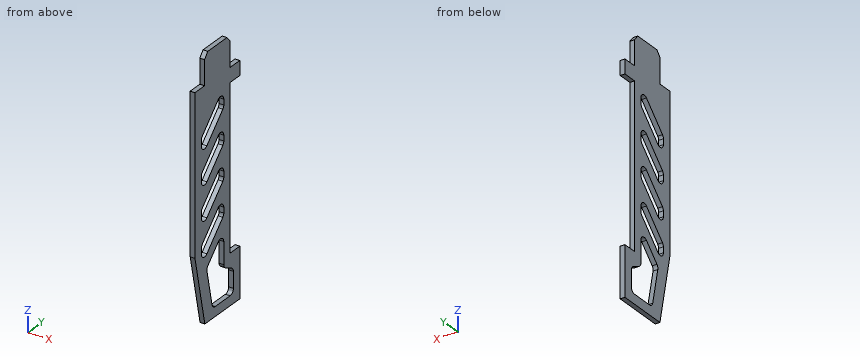
```python
from build123d import *

# Parameters (mm, degrees)
SKIZZE1_W                       = 237.5
SKIZZE1_H                       = 70
AUFSATZ_LINEAR_AUSTRAGEN1_DEPTH = 5
SCHNITT_LINEAR_AUSTRAGEN1_DEPTH = 248.651468802
SKIZZE3_W                       = 170
SKIZZE3_H                       = 15
SCHNITT_LINEAR_AUSTRAGEN2_DEPTH = 5
SCHNITT_LINEAR_AUSTRAGEN3_DEPTH = 248.651468802
VERRUNDUNG1_R                   = 5
LASCHENASE_DEPTH                = 5


with BuildPart() as part:
    # Skizze1 → Aufsatz-Linear austragen1 (new body)
    with BuildSketch(Plane(origin=(0, 0, 0), x_dir=(0, 0, -1), z_dir=(1, 0, 0))):
        with Locations((118.75, 35)):
            Rectangle(SKIZZE1_W, SKIZZE1_H)
    extrude(amount=AUFSATZ_LINEAR_AUSTRAGEN1_DEPTH)

    # Skizze2 → Schnitt-Linear austragen1 (cut, through all)
    with BuildSketch(Plane(origin=(5, 0, 0), x_dir=(0, 0, -1), z_dir=(1, 0, 0))):
        Polygon((165, 0), (237.5, 15.410350721), (237.5, 0), align=None)
    extrude(amount=-SCHNITT_LINEAR_AUSTRAGEN1_DEPTH, mode=Mode.SUBTRACT)

    # Skizze3 → Schnitt-Linear austragen2 (cut)
    with BuildSketch(Plane(origin=(5, 0, 0), x_dir=(0, 0, -1), z_dir=(1, 0, 0))):
        with Locations((100, 62.5)):
            Rectangle(SKIZZE3_W, SKIZZE3_H)
    extrude(amount=-SCHNITT_LINEAR_AUSTRAGEN2_DEPTH, mode=Mode.SUBTRACT)

    # Skizze4 → Schnitt-Linear austragen3 (cut, through all)
    with BuildSketch(Plane(origin=(5, 0, 0), x_dir=(0, 0, -1), z_dir=(1, 0, 0))):
        Polygon((15, 45), (50, 10), (70, 10), (35, 45), align=None)
        Polygon((50.884510848, 45), (70.884510848, 45), (105.884510848, 10), (85.884510848, 10), align=None)
        Polygon((86.769021696, 45), (106.769021696, 45), (141.769021696, 10), (121.769021696, 10), align=None)
        Polygon((122.653532545, 45), (142.653532545, 45), (177.653532545, 10), (157.653532545, 10), align=None)
        Polygon((227.5, 60), (227.5, 27.5), (183.622185543, 18.173482625), (156.795668168, 45), (195, 45), (202.5, 60), align=None)
    extrude(amount=-SCHNITT_LINEAR_AUSTRAGEN3_DEPTH, mode=Mode.SUBTRACT)

    # Verrundung1
    verrundung1_edges = [part.edges().sort_by_distance(p)[0] for p in [
        (2.5, 60, -202.5),
        (2.5, 60, -227.5),
        (2.5, 27.5, -227.5),
        (2.5, 18.173482625, -183.622185543),
        (2.5, 45, -156.795668168),
        (2.5, 45, -195),
        (2.5, 10, -85.884510848),
        (2.5, 45, -50.884510848),
        (2.5, 45, -70.884510848),
        (2.5, 10, -105.884510848),
        (2.5, 10, -157.653532545),
        (2.5, 45, -122.653532545),
        (2.5, 45, -142.653532545),
        (2.5, 10, -177.653532545),
        (2.5, 10, -121.769021696),
        (2.5, 45, -86.769021696),
        (2.5, 45, -106.769021696),
        (2.5, 10, -141.769021696),
        (2.5, 45, -15),
        (2.5, 45, -35),
        (2.5, 10, -70),
        (2.5, 10, -50),
    ]]
    fillet(verrundung1_edges, radius=VERRUNDUNG1_R)

    # Skizze5 → LascheNase (add)
    with BuildSketch(Plane(origin=(5, 0, 0), x_dir=(0, 0, -1), z_dir=(1, 0, 0))):
        Polygon((0, 55), (-26, 55), (-32, 49.965402213), (-32, 20.034597787), (-26, 15), (0, 15), align=None)
    extrude(amount=-LASCHENASE_DEPTH)


solid = part.part
```
Can you work these out from the model? Positions are in its coordinate system, mm. Coordinates: 2 decimals unless noted, no trailing zeros. Loops run counter-clockwise (first coordinate to the right, second up) from the corner with the lowest first, then second, coordinate; pieces in that order, holes last. Notation, with made-up numbers: M 41,-35 L 93,-35 A29 cw 93,1 Z; hole C 33,-7.75 d3. An arc over 180 degrees is marked long. Put each result on its own line as item: value. Start each with the question number.
(1) Imagine slicing it at C-C on x = 3.4. Give the number of separate pieces and of enclosed holes in the cut face, and give its area (3 significant figures).
(2) Imagine slicing it at A-A on z = -82. List the corners of the cut face in (x, y) for me, and give its area (3 significant figures).
(3) I need wall thicknesses on probe 1 along Z at (x, y) = (2.65, 36); probe 2 along Z at (x, y) = (1.55, 33); probe 3 along Z at (x, y) = (4.8, 65). Which ranges of each line are inside material? Lowest first, please.
(4) Imagine slicing it at B-B on y = 40.5. List the corners of the cut face in (x, z) for me.
(5) Will these pins go through, and if not, where does the flat tip stop? pin 1 Ø1.5 at (x, z) = (3, -66.5) entering from -Y; pin 2 Ø1.5 at (x, z) = (2.5, -54) entering from +Y; pin 3 Ø2.5 at (x, y) = (3.5, 64.5) entering from +Z; pin 4 Ø1.5 at (x, z) = (2.5, 8) entering from -Y.
Worked answers:
1. separate pieces: 1
1. enclosed holes: 5
1. area: 10,500 mm2
2. outline: M 0,0 L 5,0 L 5,13.88 L 0,13.88 Z; M 0,33.88 L 5,33.88 L 5,55 L 0,55 Z
2. area: 175 mm2
3. probe 1: z = -237.5 to -227.5, -165.8 to -151.65, -131.65 to -115.77, -95.77 to -79.88, -59.88 to -44, -24 to 32
3. probe 2: z = -237.5 to -227.5, -168.8 to -154.65, -134.65 to -118.77, -98.77 to -82.88, -62.88 to -47, -27 to 32
3. probe 3: z = -237.5 to -185, -15 to 0
4. outline: M 0,-237.5 L 5,-237.5 L 5,-227.5 L 0,-227.5 Z; M 0,-163.89 L 5,-163.89 L 5,-147.15 L 0,-147.15 Z; M 0,-129.75 L 5,-129.75 L 5,-111.27 L 0,-111.27 Z; M 0,-93.87 L 5,-93.87 L 5,-75.38 L 0,-75.38 Z; M 0,-57.98 L 5,-57.98 L 5,-39.5 L 0,-39.5 Z; M 0,-22.1 L 5,-22.1 L 5,32 L 0,32 Z
5. pin 1: stops at y = 0
5. pin 2: stops at y = 55
5. pin 3: stops at z = 0
5. pin 4: stops at y = 15
